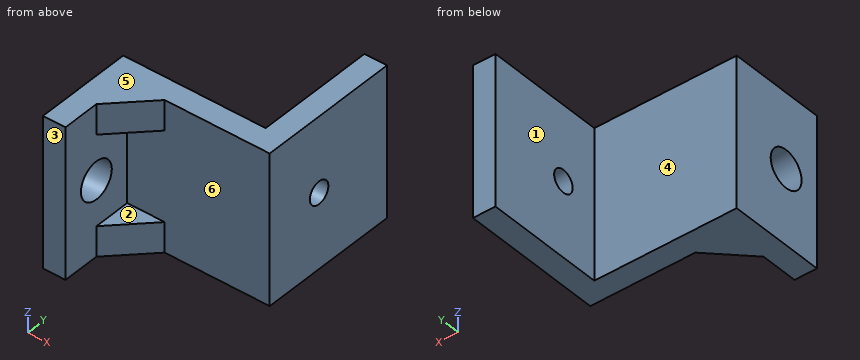
Autodesk Inventor part; units mm, degrees
ref_plane "YZ Plane" through (0, 0, 0) normal (1, 0, 0) x (0, 1, 0)
ref_plane "XZ Plane" through (0, 0, 0) normal (0, 1, 0) x (-1, 0, 0)
ref_plane "XY Plane" through (0, 0, 0) normal (0, 0, 1) x (1, 0, 0)
sketch "Sketch1" plane through (0, 0, 0) normal (0, 0, 1) x (1, 0, 0)
  line L0 (0, 0) -> (22, 0)
  line L1 (22, 0) -> (22, -19)
  line L2 (22, -19) -> (0, -19)
  line L3 (0, -19) -> (0, 0)
  line L4 (3, 0) -> (19, 0)
  line L5 (19, 0) -> (19, -16)
  line L6 (19, -16) -> (3, -16)
  line L7 (3, -16) -> (3, 0)
  dimension "d0" = 22
  dimension "d1" = 19
  dimension "d2" = 3
  dimension "d3" = 3
  dimension "d4" = 3
extrude "Extrusion1" add sketch "Sketch1" along normal blind 20 contours L0 L7 L6 L5 L1 L2 L3
sketch "Sketch4" plane through (3, -16, 0) normal (1, 0, 0) x (0, 0, -1)
  line L0 (-20, 0) -> (-20, 16)
  line L1 (0, 0) -> (-20, 0)
  line L2 (-20, 0) -> (-20, 16)
  line L3 (-20, 16) -> (0, 16)
  line L4 (0, 16) -> (0, 0)
extrude "Extrusion4" cut sketch "Sketch4" against normal through all
sketch "Sketch5" plane through (0, 0, 0) normal (0, 0, -1) x (-1, 0, 0)
  line L0 (0, -19) -> (-22, -19)
  line L1 (0, -19) -> (-3, -19)
  line L2 (-3, -19) -> (-3, -29)
  line L3 (-3, -29) -> (0, -29)
  line L4 (0, -29) -> (0, -19)
  point P0 (0, 0)
  dimension "d17" = 3
  dimension "d18" = 10
extrude "Extrusion5" add sketch "Sketch5" against normal blind 20
sketch "Sketch6" plane through (3, -29, 0) normal (1, 0, 0) x (0, 0, -1)
  line L0 (0, 10) -> (-20, 10)
  line L1 (0, 10) -> (0, 0)
  circle A0 centre (-10, 5) radius 2.5
  point P0 (0, 29)
  dimension "d21" = 5
  dimension "d22" = 10
  dimension "d23" = 5
extrude "Extrusion6" cut sketch "Sketch6" against normal through all
sketch "Sketch7" plane through (0, 0, 0) normal (0, 0, -1) x (-1, 0, 0)
  line L0 (-3, -19) -> (-22, -19)
  line L1 (-3, -29) -> (-3, -19)
  line L2 (-8, -19) -> (-3, -24)
  point P0 (0, 0)
  dimension "d26" = 5
  dimension "d27" = 5
extrude "Extrusion7" add sketch "Sketch7" against normal blind 4
sketch "Sketch8" plane through (0, 0, 20) normal (0, 0, 1) x (1, 0, 0)
  line L0 (3, -19) -> (22, -19)
  line L1 (3, -29) -> (3, -19)
  line L2 (8, -19) -> (3, -24)
  point P0 (0, 0)
  dimension "d30" = 5
  dimension "d31" = 5
extrude "Extrusion8" add sketch "Sketch8" against normal blind 4
sketch "Sketch9" plane through (19, -16, 0) normal (-1, 0, 0) x (0, 0, 1)
  line L0 (0, 16) -> (0, 0)
  line L1 (0, 0) -> (20, 0)
  circle A0 centre (10, 5) radius 1.5
  dimension "d34" = 10
  dimension "d35" = 5
  dimension "d36" = 3
extrude "Extrusion9" cut sketch "Sketch9" against normal through all
equation "\"d3\" = d2"
equation "\"d4\" = d2"
equation "\"d27\" = d26"
equation "\"d30\" = d26"
equation "\"d31\" = d30"
properties part number "LED strip mount v02"
Check sheet for the modelled part. Datum: model origin and axes. Units: mm. Face numbers are marked on the shaded views. A direction names the side the tool comes from. Give positions to 0.01 mm unless a question says otherwise; leave off trailing zeros. Order: outer loops, then holes, each group sorted by start corner. A loop starts at its lowest first (then second) coordinate and runs counter-clockwise, first axis right, second up. Notation, with made-up numbers: M 36.5,-19.75 L 48.5,-19.75 A22 cw 48.5,-2.75 Z; hole C 25.5,41 d1. An arc over 180 degrees is marked long. Answer in a Markdown table with one row per item. Add a question column.
Q1. Sectioned sample at A-A, the plane z = 10. Record the boundary of the cut face in (x, y), and give its area (3 significant figures).
Q2. Gauge pin test, flat ends, axial feed: pin 1 Ø3 at (y, z) = (-23, 7.5) entering from +X; pin 2 Ø1.5 at (x, z) = (11, 9.5) entering from +Y; pin 3 Ø2 at (x, z) = (13.5, 5.5) entering from -Y. Record the tip position at first contact, or that the pin passes through.
Q3. Access from +Z, -Z, +X, -X, +Y, -Y to the whole of each face (thin tool, end or side, straight path). Record for the marked faces 1, 2 and 3.
Q4. Thickness scan on L1, parallel to Y at x = 2.3, z = 10; L2, parallel to Y at x = 20.1, z = 10; L3, parallel to X at y = -27, z = 17. Record the ranges inside material, lowest first.
Q5. Sectioned sample at B-B, the plane x = 1.5. Record the boundary of the cut face in (y, z).
Q6. Sectioned sample at C-C, the plane y = -11. Record the boundary of the cut face in (x, z), and give its area (3 significant figures).
Q7. Release check for a two-part mould opening along Z. For the marked faces 4, 5 and 6 record: released by +Z, released by -Z, zero draft, split by the parting line, or undercut.
Q8. Sectioned sample at D-D, the plane x = 6.25. Record the boundary of the cut face in (y, z).
Verdict:
| question | item | result |
|---|---|---|
| 1 | outline | M 0,-29 L 3,-29 L 3,-26.5 L 0,-26.5 Z; M 0,-21.5 L 3,-21.5 L 3,-19 L 22,-19 L 22,-12.5 L 19,-12.5 L 19,-16 L 0,-16 Z; M 19,-9.5 L 22,-9.5 L 22,0 L 19,0 Z |
| 1 | area | 120 mm² |
| 2 | pin 1 | x = 3 |
| 2 | pin 2 | y = -16 |
| 2 | pin 3 | y = -19 |
| 3 | face 1 | +Z, -Z, -X, +Y |
| 3 | face 2 | +X, -Y |
| 3 | face 3 | +Z, -Z, +X, -X, -Y |
| 4 | L1 | -29 to -26.5, -21.5 to -16 |
| 4 | L2 | -19 to -12.5, -9.5 to 0 |
| 4 | L3 | 0 to 3 |
| 5 | outline | M -29,0 L -16,0 L -16,20 L -29,20 Z; hole C -24,10 d5 |
| 6 | outline | M 19,0 L 22,0 L 22,8.5 L 19,8.5 Z; M 19,11.5 L 22,11.5 L 22,20 L 19,20 Z |
| 6 | area | 51.0 mm² |
| 7 | face 4 | zero draft |
| 7 | face 5 | released by +Z |
| 7 | face 6 | undercut |
| 8 | outline | M -20.75,0 L -16,0 L -16,20 L -20.75,20 L -20.75,16 L -19,16 L -19,4 L -20.75,4 Z |
